```python
from build123d import *

# Parameters (mm, degrees)
BOSS_EXTRUDE1_DEPTH = 6
SKETCH2_R           = 6.5
BOSS_EXTRUDE2_DEPTH = 16
SKETCH3_R           = 2.409375482
CUT_EXTRUDE1_DEPTH  = 2.5


with BuildPart() as part:
    # Sketch1 → Boss-Extrude1 (new body)
    with BuildSketch(Plane(origin=(0, 0, 0), x_dir=(0, 0, -1), z_dir=(1, 0, 0))):
        with BuildLine():
            Line((-10, 0), (-15, 0))
            ThreePointArc((-15, 0), (-22.071067812, -2.928932188), (-25, -10))
            Line((-25, -10), (-25, -50))
            Line((-25, -50), (0, -50))
            Line((0, -50), (0, -10))
            ThreePointArc((0, -10), (-2.928932188, -2.928932188), (-10, 0))
        make_face()
    extrude(amount=BOSS_EXTRUDE1_DEPTH)

    # Sketch2 → Boss-Extrude2 (add)
    with BuildSketch(Plane(origin=(6, 0, 0), x_dir=(0, 0, -1), z_dir=(1, 0, 0))):
        with Locations(Location((-12.165364516, -9.941403235, 0), (0, 0, 180))):
            Circle(SKETCH2_R)
    extrude(amount=BOSS_EXTRUDE2_DEPTH)

    # Sketch3 → Cut-Extrude1 (cut)
    with BuildSketch(Plane.ZY):
        with Locations((12.90156258, -42.802607731)):
            Circle(SKETCH3_R)
    extrude(amount=-CUT_EXTRUDE1_DEPTH, mode=Mode.SUBTRACT)


solid = part.part
```
CAD build for the part. Positions are in the model's coordinates, mm. A direction names the side the tool comes from. Coordinates: 2 decimals unless noted, no trailing zeros. Order: outer loops, then holes, each group sorted by start corner. A loop starts at its lowest first (then second) coordinate and runs counter-clockwise, first axis right, second up. Notation, with made-up numbers: (5, 29.5) -> (29, 29.5) arc R14 cw to (29, 53.5) -> close; hole circle Ø10 at (-6.5, -32). An arc over 180 degrees is marked (long way). Use one line per item in the form item = value. Start each with the question number.
1) Band-saw the part on D-D on z = 8.5. Give the cut face in (x, y).
2) Tool access for faces 5 (the flat face through (3, -30, 25)), 6 (the cylindrical face through (13.89, -14.33, 7.37)): list every direction of +Z, -Z, +X, -X, +Y, -Y with a clear straight run to the whole face (end or side of a thin tool).
3) Band-saw the part on A-A on x = 3.5. Give the cut face in (y, z).
4) Band-saw the part on B-B on z = 11.25. Give the cut face in (x, y), then the cut area to 3 significant figures.
5) Drop flat-ended pins along their axis: pin 1 (1 mm diameter, centred on x = 11.5, z = 12, fed in from -Y); pin 2 (1.5 mm diameter, centred on x = 15, z = 20.5, fed in from -Y); pin 3 (12 mm diameter, centred on y = -38.5, z = 7.5, fed in from -X); pin 4 (8 mm diameter, centred on y = -44, z = 16.5, fed in from +X). Give the stop position or say it passes through.
6) Drill centre lines: L1, parallel to X at y = -31.5, z = 3; L2, parallel to X at y = -44, z = 13.25; L3, parallel to Y at x = 19.5, z = 11.25. Where is each one in solid material? Low to high. Write a range as [from, to].
7) Band-saw the part on C-C on y = -37.5. Give the cut face in (x, z).
8) Pull direction Y, two halves, no side cores. Call faces 1 (the cylindrical face through (1.232, -40.414, 12.588)), 2 (the flat face through (3, -30, 0)), 3 (the flat face through (2.5, -43, 13)), 4 (the cylindrical face through (2.96, -3.01, 2.85)): +Y half, -Y half, draft (parallel to the pull), parting line (faces both ways), or undercut.
Entries:
q1.outline = (0, -50) -> (6, -50) -> (6, -15.31) -> (22, -15.31) -> (22, -4.57) -> (6, -4.57) -> (6, -0.11) -> (0, -0.11) -> close
q2.face_5 = +Z, +X, -X, +Y, -Y
q2.face_6 = +X
q3.outline = (-50, 0) -> (-10, 0) arc R10 ccw to (0, 10) -> (0, 15) arc R10 ccw to (-10, 25) -> (-50, 25) -> close
q4.outline = (0, -50) -> (6, -50) -> (6, -16.38) -> (22, -16.38) -> (22, -3.51) -> (6, -3.51) -> (6, 0) -> (0, 0) -> (0, -41.05) -> (2.5, -41.05) -> (2.5, -44.56) -> (0, -44.56) -> close
q4.area = 497 mm2
q5.pin_1 = -16.44
q5.pin_2 = through
q5.pin_3 = 0
q5.pin_4 = 6
q6.L1 = [0, 6]
q6.L2 = [2.5, 6]
q6.L3 = [-16.38, -3.51]
q7.outline = (0, 0) -> (6, 0) -> (6, 25) -> (0, 25) -> close
q8.face_1 = undercut
q8.face_2 = draft
q8.face_3 = undercut
q8.face_4 = +Y half
